from build123d import *

# Parameters (mm, degrees)
F0_R     = 152.5
F0_R_2   = 7.5
F0_R_3   = 30
F1_DEPTH = 10
F2_R     = 147.266784
F2_R_2   = 141.252776
F3_DEPTH = 40
F4_R     = 39
F5_DEPTH = 5


with BuildPart() as f1:
    # F0 (on Front) → F1 (new body)
    with BuildSketch(Plane.XZ):
        Circle(F0_R)
        with BuildLine():
            ThreePointArc((-1.5, -134.491635), (-4.599609, -137.423046), (-7.496269, -134.290938))
            Line((-7.496269, -134.290938), (-6.733122, -100.082887))
            ThreePointArc((-6.733122, -100.082887), (-3.700411, -97.149984), (-0.733868, -100.149798))
            ThreePointArc((-0.733868, -100.149798), (-0.734614, -100.216708), (-0.736853, -100.283585))
            Line((-0.736853, -100.283585), (-1.5, -134.491635))
        make_face(mode=Mode.SUBTRACT)
        with BuildLine():
            ThreePointArc((-117.223173, -65.94678), (-121.311653, -64.728145), (-120.047498, -60.653509))
            Line((-120.047498, -60.653509), (-90.040884, -44.210389))
            ThreePointArc((-90.040884, -44.210389), (-85.98456, -45.370342), (-87.099203, -49.43935))
            ThreePointArc((-87.099203, -49.43935), (-87.157522, -49.472159), (-87.216559, -49.503659))
            Line((-87.216559, -49.503659), (-117.223173, -65.94678))
        make_face(mode=Mode.SUBTRACT)
        with Locations((-42.435245, -24.5)):
            Circle(F0_R_2, mode=Mode.SUBTRACT)
        with Locations((0, -49)):
            Circle(F0_R_2, mode=Mode.SUBTRACT)
        with Locations((42.435245, -24.5)):
            Circle(F0_R_2, mode=Mode.SUBTRACT)
        with BuildLine():
            ThreePointArc((115.723173, -68.544856), (116.712045, -72.694901), (112.551229, -73.637428))
            Line((112.551229, -73.637428), (83.307762, -55.872498))
            ThreePointArc((83.307762, -55.872498), (82.284149, -51.779642), (86.365335, -50.710447))
            ThreePointArc((86.365335, -50.710447), (86.422908, -50.744549), (86.479706, -50.779926))
            Line((86.479706, -50.779926), (115.723173, -68.544856))
        make_face(mode=Mode.SUBTRACT)
        with BuildLine():
            ThreePointArc((-115.723173, 68.544856), (-116.712045, 72.694901), (-112.551229, 73.637428))
            Line((-112.551229, 73.637428), (-83.307762, 55.872498))
            ThreePointArc((-83.307762, 55.872498), (-82.284149, 51.779642), (-86.365335, 50.710447))
            ThreePointArc((-86.365335, 50.710447), (-86.422908, 50.744549), (-86.479706, 50.779926))
            Line((-86.479706, 50.779926), (-115.723173, 68.544856))
        make_face(mode=Mode.SUBTRACT)
        with Locations((-42.435245, 24.5)):
            Circle(F0_R_2, mode=Mode.SUBTRACT)
        Circle(F0_R_3, mode=Mode.SUBTRACT)
        with Locations((42.435245, 24.5)):
            Circle(F0_R_2, mode=Mode.SUBTRACT)
        with Locations((0, 49)):
            Circle(F0_R_2, mode=Mode.SUBTRACT)
        with BuildLine():
            ThreePointArc((117.223173, 65.94678), (121.311653, 64.728145), (120.047498, 60.653509))
            Line((120.047498, 60.653509), (90.040884, 44.210389))
            ThreePointArc((90.040884, 44.210389), (85.98456, 45.370342), (87.099203, 49.43935))
            ThreePointArc((87.099203, 49.43935), (87.157522, 49.472159), (87.216559, 49.503659))
            Line((87.216559, 49.503659), (117.223173, 65.94678))
        make_face(mode=Mode.SUBTRACT)
        with BuildLine():
            ThreePointArc((1.5, 134.491635), (4.599609, 137.423046), (7.496269, 134.290938))
            Line((7.496269, 134.290938), (6.733122, 100.082887))
            ThreePointArc((6.733122, 100.082887), (3.700411, 97.149984), (0.733868, 100.149798))
            ThreePointArc((0.733868, 100.149798), (0.734614, 100.216708), (0.736853, 100.283585))
            Line((0.736853, 100.283585), (1.5, 134.491635))
        make_face(mode=Mode.SUBTRACT)
    extrude(amount=F1_DEPTH)

    # F2 (on face) → F3 (join)
    with BuildSketch(Plane(origin=(0, 0, 0), x_dir=(-1, 0, 0), z_dir=(0, 1, 0))):
        Circle(F2_R)
        Circle(F2_R_2, mode=Mode.SUBTRACT)
    extrude(amount=F3_DEPTH)

    # F4 (on face) → F5 (cut)
    with BuildSketch(Plane(origin=(0, 0, 0), x_dir=(-1, 0, 0), z_dir=(0, 1, 0))):
        Circle(F4_R)
    extrude(amount=-F5_DEPTH, mode=Mode.SUBTRACT)


solid = f1.part
Design review of the part built by this model. Coordinates are the model's own, in mm. A direction names the side the tool comes from. Give positions to 0.01 mm unless a question says otherwise; leave off trailing zeros. Order: outer loops, then holes, each group sorted by start corner. A loop starts at its lowest first (then second) coordinate and runs counter-clockwise, first axis right, second up.
1. For pin 1 Ø17 at (x, z) = (-42.44, 24.5) entering from +Y; pin 2 Ø5 at (x, y) = (-119, 11) entering from +Z; pin 3 Ø12 at (x, z) = (-42.44, -24.5) entering from -Y; pin 4 Ø4 at (x, y) = (-73, 17) entering from +Z, all flat-tipped, find the tip position at first contact; note any pin that passes through.
Solution:
pin 1: stops at y = 0
pin 2: stops at z = 90.08
pin 3: passes through
pin 4: stops at z = 129.02
2. Add section C-C, the plane y = 24. State the section outline as (x, z) points.
Solution:
outline: circle Ø294.53 at (0, 0); hole circle Ø282.51 at (0, 0)
3. Add section A-A, the plane z = 0. State the section outline as (x, y) points, then the cut area to 3 significant figures.
Solution:
outline: (-152.5, -10) - (-30, -10) - (-30, -5) - (-39, -5) - (-39, 0) - (-141.25, 0) - (-141.25, 40) - (-147.27, 40) - (-147.27, 0) - (-152.5, 0) - close; (30, -10) - (152.5, -10) - (152.5, 0) - (147.27, 0) - (147.27, 40) - (141.25, 40) - (141.25, 0) - (39, 0) - (39, -5) - (30, -5) - close
area: 2,840 mm2
4. To check wall thickness, follow L1, parallel to Z at x = 0, y = -3.75; L2, parallel to Z at x = 0, y = -6; L3, parallel to Z at x = -111.5, y = -1. State the ranges of each line that lie inside material, in increasing order.
Solution:
L1: z = -152.5 to -56.5, -41.5 to -39, 39 to 41.5, 56.5 to 152.5
L2: z = -152.5 to -56.5, -41.5 to -30, 30 to 41.5, 56.5 to 152.5
L3: z = -104.04 to -62.81, -55.97 to 65.98, 73 to 104.04
5. Add section B-B, the plane x = 45. State the section outline as (y, z) points.
Solution:
outline: (-10, -145.71) - (0, -145.71) - (0, -140.22) - (40, -140.22) - (40, -133.89) - (0, -133.89) - (0, -31.55) - (-10, -31.55) - close; (-10, -17.45) - (0, -17.45) - (0, 17.45) - (-10, 17.45) - close; (-10, 31.55) - (0, 31.55) - (0, 133.89) - (40, 133.89) - (40, 140.22) - (0, 140.22) - (0, 145.71) - (-10, 145.71) - close
6. Add section D-D, the plane x = -26. State the section outline as (y, z) points.
Solution:
outline: (-10, -150.27) - (0, -150.27) - (0, -144.95) - (40, -144.95) - (40, -138.84) - (0, -138.84) - (0, -29.07) - (-5, -29.07) - (-5, -14.97) - (-10, -14.97) - close; (-10, 14.97) - (-5, 14.97) - (-5, 29.07) - (0, 29.07) - (0, 138.84) - (40, 138.84) - (40, 144.95) - (0, 144.95) - (0, 150.27) - (-10, 150.27) - close
7. Mouldability with a two-part tool opening along X and no side actions: class faces 4 (the cylindrical face through (31.925, 19.72, -143.765)), 5 (the cylindrical face through (-1.63, -4.93, 41.68)), 6 (the flat face through (32, -10, 2)), 7 (the cylindrical face through (-1.63, -4.93, -56.32)) as +X half, -X half, draft (parallel to the pull), parting line (faces both ways), or undercut.
Solution:
face 4: parting line
face 5: undercut
face 6: draft
face 7: undercut
8. Tool access review of faces 1 (the cylindrical face through (5.077, -2.465, 38.668)), 2 (the flat face through (-10.2, 40, -141.1)), 3 (the flat face through (100.9, -4.93, -59.54)): name each direction out of +Z, -Z, +X, -X, +Y, -Y from which nothing blocks a thin tool from reaching the whole face with its end or side.
Solution:
face 1: +Y
face 2: +Z, -Z, +X, -X, +Y
face 3: +Y, -Y
